For this review, take the finished solid that the model builds, in its own axes (mm). A direction names the side the tool comes from. Coordinates: 2 decimals unless noted, no trailing zeros. Order: outer loops, then holes, each group sorted by start corner. A loop starts at its lowest first (then second) coordinate and runs counter-clockwise, first axis right, second up. Notation, with made-up numbers: (45, 46.25) -> (69, 46.25) arc R7 ccw to (69, 54.25) -> close; hole circle Ø6 at (55, 88.5). An arc over 180 degrees is marked (long way). Answer as a JSON object with one key per item and string values. Group by question number.
1) Add section B-B, the plane z = 0. Write out the cut boundary in (x, y).
2) Add section D-D, the plane y = 4.25. Write out the cut boundary in (x, z), then the cut area to 3 significant figures.
3) Draft analysis for pull direction X (two halves, no side actions). For faces 1 (the cylindrical face through (-12.571, 5.07, -4.654)), 2 (the cylindrical face through (18.72, 5.07, 8.29)), 3 (the flat face through (0, 5, -9.5)), state which applies: +X half, -X half, draft (parallel to the pull), parting line (faces both ways), or undercut.
4) Add section C-C, the plane x = 15. Write out the cut boundary in (y, z), then the cut area to 3 significant figures.
5) Wall thickness on L1, parallel to Z at x = 15, y = 3.75; L2, parallel to Z at x = -15, y = 8.45; L3, parallel to Z at x = -3, y = 3: over which ranges is each line inside the solid? List them lowest first.
6) Add section A-A, the plane x = -4. Write out the cut boundary in (y, z).
7) Machinability: for faces 4 (the flat face through (0, 10, -9)), 5 (the cylindrical face through (17.32, 5.07, 6.86)), 6 (the flat face through (16.4, 7, 1.4)), which of the approach directions +Z, -Z, +X, -X, +Y, -Y give a long, thin tool a straight path to every point of the face, cutting with its end or side? Answer none if there is none.
8) For pin 1 (1 mm diameter, centred on x = 13, z = 0, fed in from +Y), flat-tipped, find the tip position at first contact; note if it passes through.
from build123d import *

# Parameters (mm, degrees)
SKETCH1_W                      = 40
SKETCH1_H                      = 19
SKETCH1_W_2                    = 36
SKETCH1_H_2                    = 15
BOSS_EXTRUDE1_DEPTH            = 10
FILLET1_R                      = 4.25
BOSS_EXTRUDE2_START            = 10
BOSS_EXTRUDE2_DEPTH            = 10
CBORE_FOR_M3_SHCS1_D           = 3.6
CBORE_FOR_M3_SHCS1_CBORE_D     = 6.5
CBORE_FOR_M3_SHCS1_CBORE_DEPTH = 3
CUT_EXTRUDE1_DEPTH             = 25.295061227
FILLET2_R                      = 2


with BuildPart() as part:
    # Sketch1 → Boss-Extrude1 (new body)
    with BuildSketch(Plane(origin=(0, 0, 0), x_dir=(1, 0, 0), z_dir=(0, 1, 0))):
        Rectangle(SKETCH1_W, SKETCH1_H)
        Rectangle(SKETCH1_W_2, SKETCH1_H_2, mode=Mode.SUBTRACT)
    extrude(amount=BOSS_EXTRUDE1_DEPTH)

    # Fillet1
    fillet1_edges = [part.edges().sort_by_distance(p)[0] for p in [
        (-18, 5, -7.5),
        (-18, 5, 7.5),
        (18, 5, 7.5),
        (18, 5, -7.5),
        (20, 5, 9.5),
        (-20, 5, 9.5),
        (-20, 5, -9.5),
        (20, 5, -9.5),
    ]]
    fillet(fillet1_edges, radius=FILLET1_R)

    # Sketch2 → Boss-Extrude2 (add)
    with BuildSketch(Plane(origin=(0, 0, 0), x_dir=(1, 0, 0), z_dir=(0, 1, 0)).offset(BOSS_EXTRUDE2_START)):
        with BuildLine():
            Line((18, -3.25), (18, 3.25))
            ThreePointArc((18, 3.25), (16.75520382, 6.25520382), (13.75, 7.5))
            Line((13.75, 7.5), (10, 7.5))
            Line((10, 7.5), (10, -7.5))
            Line((10, -7.5), (13.75, -7.5))
            ThreePointArc((13.75, -7.5), (16.75520382, -6.25520382), (18, -3.25))
        make_face()
        with BuildLine():
            Line((-13.75, -7.5), (-10, -7.5))
            Line((-10, -7.5), (-10, 7.5))
            Line((-10, 7.5), (-13.75, 7.5))
            ThreePointArc((-13.75, 7.5), (-16.75520382, 6.25520382), (-18, 3.25))
            Line((-18, 3.25), (-18, -3.25))
            ThreePointArc((-18, -3.25), (-16.75520382, -6.25520382), (-13.75, -7.5))
        make_face()
    extrude(amount=-BOSS_EXTRUDE2_DEPTH)

    # CBORE for M3 SHCS1 (through all)
    with Locations(Plane(origin=(0, 10, 0), x_dir=(1, 0, 0), z_dir=(0, 1, 0))):
        with Locations((-15, 0), (15, 0)):
            CounterBoreHole(CBORE_FOR_M3_SHCS1_D / 2, CBORE_FOR_M3_SHCS1_CBORE_D / 2, CBORE_FOR_M3_SHCS1_CBORE_DEPTH)

    # Sketch5 → Cut-Extrude1 (cut, through all)
    with BuildSketch(Plane(origin=(0, 10, 0), x_dir=(1, 0, 0), z_dir=(0, 1, 0))):
        with BuildLine():
            Line((15.75, 7.5), (-15.75, 7.5))
            ThreePointArc((-15.75, 7.5), (-17.340990258, 6.840990258), (-18, 5.25))
            Line((-18, 5.25), (-18, 4.308421985))
            ThreePointArc((-18, 4.308421985), (-9.75, 0), (-18, -4.308421985))
            Line((-18, -4.308421985), (-18, -5.25))
            ThreePointArc((-18, -5.25), (-17.340990258, -6.840990258), (-15.75, -7.5))
            Line((-15.75, -7.5), (15.75, -7.5))
            ThreePointArc((15.75, -7.5), (17.340990258, -6.840990258), (18, -5.25))
            Line((18, -5.25), (18, -4.308421985))
            ThreePointArc((18, -4.308421985), (9.75, 0), (18, 4.308421985))
            Line((18, 4.308421985), (18, 5.25))
            ThreePointArc((18, 5.25), (17.340990258, 6.840990258), (15.75, 7.5))
        make_face()
    extrude(amount=-CUT_EXTRUDE1_DEPTH, mode=Mode.SUBTRACT)

    # Fillet2
    # the kernel refuses this fillet: 2 mm, written as the material it adds along each edge
    with BuildSketch(Plane(origin=(18, 10, 4.308421985), x_dir=(-0.9035715432909278, 0, 0.42843723712447174), z_dir=(0, -1, 0)), Plane(origin=(-18, 10, -4.308421985), x_dir=(0.9035715432909261, 0, -0.4284372371244754), z_dir=(0, -1, 0))) as fillet2_piece_1:
        with BuildLine():
            CenterArc((2.059110044, -1.972677796), FILLET2_R, 99.481480479, 46.397181027)
            Line((0.403407083, -0.8507831), (0.370293024, -0.828345206))
            ThreePointArc((0.370293024, -0.828345206), (0.16556068, -0.44252904), (-0.036142862, -0.017137489))
            Line((-0.036142862, -0.017137489), (0.006589152, 0.039453556))
            ThreePointArc((0.006589152, 0.039453556), (0.864826218, -0.031720787), (1.723063284, 0.039453556))
            Line((1.723063284, 0.039453556), (1.729652437, 0))
        make_face()
    extrude(amount=10)
    with BuildSketch(Plane(origin=(18, 10, -4.308421985), x_dir=(0, 0, -1), z_dir=(0, -1, 0)), Plane(origin=(-18, 10, 4.308421985), x_dir=(0, 0, 1), z_dir=(0, -1, 0))) as fillet2_piece_2:
        with BuildLine():
            CenterArc((2.664654938, -1.015384615), FILLET2_R, 149.489762594, 46.397181027)
            Line((0.741047511, -1.562864721), (0.702575363, -1.573814324))
            ThreePointArc((0.702575363, -1.573814324), (0.399185756, -0.767841995), (-0.032826072, -0.022857143))
            Line((-0.032826072, -0.022857143), (0, 0.04))
            ThreePointArc((0, 0.04), (0.470789008, 0.04), (0.907116477, 0.020307692))
            Line((0.907116477, 0.020307692), (0.941578015, 0))
        make_face()
    extrude(amount=10)


solid = part.part
Output values:
{
 "1": {"outline": "(-20, 0) -> (-16.8, 0) -> (-16.8, 7) -> (-18.25, 7) -> (-18.25, 10) -> (-20, 10) -> close; (-13.2, 0) -> (-10, 0) -> (-10, 10) -> (-11.75, 10) -> (-11.75, 7) -> (-13.2, 7) -> close; (10, 0) -> (13.2, 0) -> (13.2, 7) -> (11.75, 7) -> (11.75, 10) -> (10, 10) -> close; (16.8, 0) -> (20, 0) -> (20, 10) -> (18.25, 10) -> (18.25, 7) -> (16.8, 7) -> close"},
 "2": {"outline": "(-20, -5.25) arc R4.25 ccw to (-15.75, -9.5) -> (15.75, -9.5) arc R4.25 ccw to (20, -5.25) -> (20, 5.25) arc R4.25 ccw to (15.75, 9.5) -> (-15.75, 9.5) arc R4.25 ccw to (-20, 5.25) -> close; hole (-18, -5.25) arc R2.25 ccw to (-15.75, -7.5) -> (15.75, -7.5) arc R2.25 ccw to (18, -5.25) arc R2 ccw to (16.44, -5.05) arc R5.25 cw to (10, -1.6) -> (10, 1.6) arc R5.25 cw to (16.44, 5.05) arc R2 ccw to (18, 5.25) arc R2.25 ccw to (15.75, 7.5) -> (-15.75, 7.5) arc R2.25 ccw to (-18, 5.25) arc R2 ccw to (-16.44, 5.05) arc R5.25 cw to (-10, 1.6) -> (-10, -1.6) arc R5.25 cw to (-16.44, -5.05) arc R2 ccw to start; hole circle Ø3.6 at (-15, 0); hole circle Ø3.6 at (15, 0)", "area": "335 mm²"},
 "3": {"face 1": "undercut", "face 2": "+X half", "face 3": "draft"},
 "4": {"outline": "(0, -9.5) -> (10, -9.5) -> (10, -7.5) -> (0, -7.5) -> close; (0, -5.25) -> (10, -5.25) -> (10, -3.25) -> (7, -3.25) -> (7, -1.8) -> (0, -1.8) -> close; (0, 1.8) -> (7, 1.8) -> (7, 3.25) -> (10, 3.25) -> (10, 5.25) -> (0, 5.25) -> close; (0, 7.5) -> (10, 7.5) -> (10, 9.5) -> (0, 9.5) -> close", "area": "100 mm²"},
 "5": {"L1": "z = -9.5 to -7.5, -5.25 to -1.8, 1.8 to 5.25, 7.5 to 9.5", "L2": "z = -9.5 to -7.5, -5.25 to -3.25, 3.25 to 5.25, 7.5 to 9.5", "L3": "z = -9.5 to -7.5, 7.5 to 9.5"},
 "6": {"outline": "(0, -9.5) -> (10, -9.5) -> (10, -7.5) -> (0, -7.5) -> close; (0, 7.5) -> (10, 7.5) -> (10, 9.5) -> (0, 9.5) -> close"},
 "7": {"face 4": "+Z, -Z, +X, -X, +Y", "face 5": "+Y, -Y", "face 6": "+Y"},
 "8": {"pin 1": "stops at y = 7"}
}
